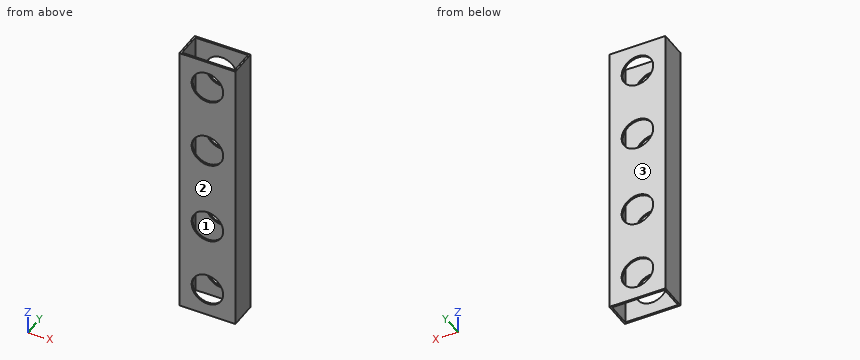
Autodesk Inventor part; units mm, degrees
ref_plane "YZ Plane" through (0, 0, 0) normal (1, 0, 0) x (0, 1, 0)
ref_plane "XZ Plane" through (0, 0, 0) normal (0, 1, 0) x (-1, 0, 0)
ref_plane "XY Plane" through (0, 0, 0) normal (0, 0, 1) x (1, 0, 0)
sketch "Sketch1" plane through (0, 0, 0) normal (0, 0, 1) x (1, 0, 0)
  line L0 (0, 0) -> (50.8, 0)
  line L1 (50.8, 0) -> (50.8, 25.4)
  line L2 (50.8, 25.4) -> (0, 25.4)
  line L3 (0, 25.4) -> (0, 0)
  dimension "d0" = 50.8
  dimension "d1" = 25.4
extrude "Extrusion1" add sketch "Sketch1" along normal blind 254
shell "Shell1" thickness 1.5875 removed faces 2 at (16.9333, 8.4667, 0) at (16.9333, 8.4667, 254)
sketch "Sketch2" plane through (0, 25.4, 0) normal (0, 1, 0) x (1, 0, 0)
  circle A0 centre (25.4, -25.4) radius 14.2875
  circle A1 centre (25.4, -228.6) radius 14.2875
  line L0 (0, -254) -> (50.8, -254)
  line L1 (50.8, 0) -> (0, 0)
  line L2 (0, 0) -> (0, -254)
  circle A2 centre (25.4, -88.9) radius 14.2875
  circle A3 centre (25.4, -165.1) radius 14.2875
  dimension "d5" = 25.4
  dimension "d6" = 25.4
  dimension "d7" = 25.4
  dimension "d8" = 25.4
  dimension "d9" = 28.575
  dimension "d12" = 25.4
  dimension "d13" = 25.4
  dimension "d14" = 76.2
  dimension "d15" = 88.9
extrude "Extrusion2" cut sketch "Sketch2" against normal through all
equation "\"d2\" = Length"
equation "\"d6\" = d5"
equation "\"d7\" = d6"
equation "\"d8\" = d5"
equation "\"d12\" = d13"
equation "\"d13\" = d8"
equation "\"Length\" = 254"
properties part number "Main body"
Can you work these out from the model? Positions are in its coordinate system, mm. Face numbers are marked on the shaded views. Round coordinates to 2 decimals unless told otherwise and drop trailing zeros. Order: outer loops, then holes, each group sorted by start corner. A loop starts at its lowest first (then second) coordinate and runs counter-clockwise, first axis right, second up. Notation, with made-up numbers: (-19.5, -5) -> (-12.5, -5) arc R7 ccw to (-12.5, 4) -> close; hole circle Ø3 at (79.5, 11.25). An arc over 180 degrees is marked (long way). Write each question's results on one line, items separated by ' | '. Start each with the question number.
Item 1: Will this pin go through, and if not, where does the flat tip stop? pin 1 (10 mm diameter, centred on x = 25, y = 4.5, fed in from +Z).
Item 2: If we section it at B-B, the plane z = 144.5: Write out the boundary of the cut face in (x, y).
Item 3: Thinking about a two-plate mould opening in Y: for the marked faces 1, 2 and 3, which applies, +Y half, -Y half, draft (parallel to the pull), parting line (faces both ways), or undercut?
Item 4: If we section it at C-C, the plane x = 4.5: Write out the boundary of the cut face in (y, z), then the cut area to 3 significant figures.
Item 5: If we section it at A-A, the plane y = 12.5: Write out the boundary of the cut face in (x, z).
Item 6: Please list where these lines run through material, in increasing order: L1, parallel to Z at x = 25.4, y = 1; L2, parallel to X at y = 6.25, z = 206; L3, parallel to X at y = 24.75, z = 165.1.
Item 7: If we section it at D-D, the plane z = 174.5: Write out the boundary of the cut face in (x, y).
Results:
1) pin 1: stops at z = 254
2) outline: (0, 0) -> (50.8, 0) -> (50.8, 25.4) -> (0, 25.4) -> close; hole (1.59, 1.59) -> (49.21, 1.59) -> (49.21, 23.81) -> (1.59, 23.81) -> close
3) face 1: undercut | face 2: -Y half | face 3: +Y half
4) outline: (0, 0) -> (1.59, 0) -> (1.59, 254) -> (0, 254) -> close; (23.81, 0) -> (25.4, 0) -> (25.4, 254) -> (23.81, 254) -> close | area: 806 mm2
5) outline: (0, 0) -> (1.59, 0) -> (1.59, 254) -> (0, 254) -> close; (49.21, 0) -> (50.8, 0) -> (50.8, 254) -> (49.21, 254) -> close
6) L1: z = 0 to 11.11, 39.69 to 74.61, 103.19 to 150.81, 179.39 to 214.31, 242.89 to 254 | L2: x = 0 to 1.59, 49.21 to 50.8 | L3: x = 0 to 11.11, 39.69 to 50.8
7) outline: (0, 0) -> (14.64, 0) -> (14.64, 1.59) -> (1.59, 1.59) -> (1.59, 23.81) -> (14.64, 23.81) -> (14.64, 25.4) -> (0, 25.4) -> close; (36.16, 0) -> (50.8, 0) -> (50.8, 25.4) -> (36.16, 25.4) -> (36.16, 23.81) -> (49.21, 23.81) -> (49.21, 1.59) -> (36.16, 1.59) -> close
